Input: part model. Units: mm. Frame: model coordinates. A direction names the side the tool comes from. Coordinates: 2 decimals unless noted, no trailing zeros. Write each loop counter-clockwise with the first axis right and the second up, starting at its lowest first coordinate (ties: lowest second). Pieces come first, ordered by that corner, then holes. Notation, with made-up numbers: M 33.25,50.5 L 83.25,50.5 A13 cw 83.25,72.5 Z; hole C -8.75,1.25 d6. An arc over 180 degrees is marked long. Use one line per item in the form item = value.
from build123d import *

# Parameters (mm, degrees)
SKETCH_1_W           = 232.8
SKETCH_1_H           = 162
SKETCH_1_R           = 72
EXTRUDE_1_DEPTH      = 4
CUT_EXTRUDE_START    = -10
CUT_EXTRUDE_2_DEPTH  = 10
EXTRUDE_2_DEPTH      = 4
CUT_EXTRUDE_3_DEPTH  = 10
SKETCH_5_R           = 1.6
CUT_EXTRUDE_4_DEPTH  = 10
SKETCH_9_R           = 1.6
CUT_EXTRUDE_5_DEPTH  = 10
SKETCH_10_R          = 1.6
CUT_EXTRUDE_6_DEPTH  = 10
SKETCH_11_R          = 1.6
CUT_EXTRUDE_7_DEPTH  = 10
CUT_EXTRUDE_8_DEPTH  = 10
FILLET_1_R           = 3
FILLET_2_R           = 1.1
FILLET_3_R           = 3
CUT_EXTRUDE_9_DEPTH  = 10
FILLET_4_R           = 3
SKETCH_14_W          = 34.4
SKETCH_14_H          = 162
CUT_EXTRUDE_10_DEPTH = 10
CUT_EXTRUDE_11_DEPTH = 10
FILLET_5_R           = 3
SKETCH_16_R          = 1.55
CUT_EXTRUDE_12_DEPTH = 10
SKETCH_17_W          = 200
SKETCH_17_H          = 10
CUT_EXTRUDE_13_DEPTH = 5
FILLET_6_R           = 3


with BuildPart() as part:
    # 草图1 → 凸台-拉伸1 (new body)
    with BuildSketch(Plane.XY):
        Rectangle(SKETCH_1_W, SKETCH_1_H)
        Circle(SKETCH_1_R, mode=Mode.SUBTRACT)
    extrude(amount=EXTRUDE_1_DEPTH)

    # 草图3 → 切除-拉伸2 (cut)
    with BuildSketch(Plane.XY.offset(4).offset(CUT_EXTRUDE_START)):
        with BuildLine():
            Line((-21.634615385, 68.67272688), (-116.4, 38.817895988))
            Line((-116.4, 38.817895988), (-116.4, -7.313954951))
            Line((-116.4, -7.313954951), (-71.680591647, 6.774421088))
            ThreePointArc((-71.680591647, 6.774421088), (-55.989124219, 45.268288781), (-21.634615385, 68.67272688))
        make_face()
    extrude(amount=CUT_EXTRUDE_2_DEPTH, mode=Mode.SUBTRACT)

    # 草图6 → 凸台-拉伸2 (add)
    with BuildSketch(Plane.XY.offset(4)):
        Polygon((-126.671662246, -16.840640315), (-116.4, -29.949880057), (-116.4, -7.313954951), (-128.474546862, -11.117913075), align=None)
        Polygon((-116.4, 38.817895988), (-116.4, 54.514482194), (-143.498585323, 36.571480592), (-141.695700708, 30.848753352), align=None)
    extrude(amount=-EXTRUDE_2_DEPTH)

    # 草图7 → 切除-拉伸3 (cut)
    with BuildSketch(Plane.XY.offset(4)):
        Polygon((-116.4, -29.949880057), (-76.4, -81), (-116.4, -81), align=None)
        Polygon((-116.4, 54.514482194), (-76.4, 81), (-116.4, 81), align=None)
    extrude(amount=-CUT_EXTRUDE_3_DEPTH, mode=Mode.SUBTRACT)

    # 草图5 → 切除-拉伸4 (cut)
    with BuildSketch(Plane.XY.offset(4)):
        with Locations((-115.25907459, -12.196774271)):
            Circle(SKETCH_5_R)
        with Locations((-131.485036128, 39.307770889)):
            Circle(SKETCH_5_R)
    extrude(amount=-CUT_EXTRUDE_4_DEPTH, mode=Mode.SUBTRACT)

    # 草图9 → 切除-拉伸5 (cut)
    with BuildSketch(Plane.XY.offset(4)):
        with Locations((-22.836538462, 72.487878374)):
            Circle(SKETCH_9_R)
        with Locations((72.487878374, 22.836538462)):
            Circle(SKETCH_9_R)
        with Locations((22.836538462, -72.487878374)):
            Circle(SKETCH_9_R)
        with Locations((-72.487878374, -22.836538462)):
            Circle(SKETCH_9_R)
    extrude(amount=-CUT_EXTRUDE_5_DEPTH, mode=Mode.SUBTRACT)

    # 草图10 → 切除-拉伸6 (cut)
    with BuildSketch(Plane.XY.offset(4)):
        with Locations((-93.229198124, 50.99070111)):
            Circle(SKETCH_10_R)
    extrude(amount=-CUT_EXTRUDE_6_DEPTH, mode=Mode.SUBTRACT)

    # 草图11 → 切除-拉伸7 (cut)
    with BuildSketch(Plane(origin=(0, 0, 0), x_dir=(-1, 0, 0), z_dir=(0, 0, -1))):
        with Locations((-35.108799147, 67.404541557)):
            Circle(SKETCH_11_R)
        with Locations((-67.404541557, -35.108799147)):
            Circle(SKETCH_11_R)
        with Locations((35.108799147, -67.404541557)):
            Circle(SKETCH_11_R)
    extrude(amount=-CUT_EXTRUDE_7_DEPTH, mode=Mode.SUBTRACT)

    # 草图12 → 切除-拉伸8 (cut)
    with BuildSketch(Plane.XY.offset(4)):
        Polygon((-93.668674526, 62.369689763), (-74.593630829, 75), (-25.836538462, 75), (-25.836538462, 72.5912113), (-90.473635724, 52.227978291), align=None)
    extrude(amount=-CUT_EXTRUDE_8_DEPTH, mode=Mode.SUBTRACT)

    # 圆角1
    # the kernel refuses this fillet: 3 mm, written as the material it adds along each edge
    with BuildSketch(Plane(origin=(-25.836538462, 75, 4), x_dir=(0, -1, 0), z_dir=(0, 0, -1)), Plane(origin=(-90.473635724, 52.227978291, 4), x_dir=(-0.3004807692307691, 0.95378787333583, 0), z_dir=(0, 0, -1))) as fillet_1_piece_1:
        with BuildLine():
            CenterArc((FILLET_1_R, FILLET_1_R), FILLET_1_R, 180, 90)
            Line((0, FILLET_1_R), (0, 0))
            Line((0, 0), (FILLET_1_R, 0))
        make_face()
    extrude(amount=4)
    with BuildSketch(Plane(origin=(-25.836538462, 72.5912113, 4), x_dir=(-0.9537878733358296, -0.30048076923076983, 0), z_dir=(0, 0, -1))) as fillet_1_piece_2:
        with BuildLine():
            CenterArc((FILLET_1_R * 0.733411747334, FILLET_1_R), FILLET_1_R, 197.486481518, 72.513518482)
            Line((-FILLET_1_R * 0.220376126002, FILLET_1_R * 0.699519230769), (0, 0))
            Line((0, 0), (FILLET_1_R * 0.733411747334, 0))
        make_face()
    extrude(amount=4)
    with BuildSketch(Plane(origin=(-93.668674526, 62.369689763, 4), x_dir=(0.3004807692307694, -0.95378787333583, 0), z_dir=(0, 0, -1))) as fillet_1_piece_3:
        with BuildLine():
            CenterArc((FILLET_1_R * 0.753231578374, -FILLET_1_R), FILLET_1_R, 90, 73.976427328)
            Line((-FILLET_1_R * 0.207916633287, -FILLET_1_R * 0.72396718452), (0, 0))
            Line((0, 0), (FILLET_1_R * 0.753231578374, 0))
        make_face()
    extrude(amount=4)
    with BuildSketch(Plane(origin=(-74.593630829, 75, 4), x_dir=(1, 0, 0), z_dir=(0, 0, -1))) as fillet_1_piece_4:
        with BuildLine():
            CenterArc((FILLET_1_R * 0.30106152849, FILLET_1_R), FILLET_1_R, 236.48994581, 33.51005419)
            Line((-FILLET_1_R * 0.251021777541, FILLET_1_R * 0.166211043968), (0, 0))
            Line((0, 0), (FILLET_1_R * 0.30106152849, 0))
        make_face()
    extrude(amount=4)

    # 圆角2
    fillet_2_edges = [part.edges().sort_by_distance(p)[0] for p in [
        (-26.180986438, 73.395723271, 2),
    ]]
    fillet(fillet_2_edges, radius=FILLET_2_R)

    # 圆角3
    fillet_3_edges = [part.edges().sort_by_distance(p)[0] for p in [
        (-71.680591647, 6.774421088, 2),
        (-76.4, -81, 2),
        (-76.4, 81, 2),
    ]]
    fillet(fillet_3_edges, radius=FILLET_3_R)

    # 草图13 → 切除-拉伸9 (cut)
    with BuildSketch(Plane.XY.offset(4)):
        with BuildLine():
            Line((-71.696957036, -36.822633688), (-92.944059946, -46.914680662))
            Line((-92.944059946, -46.914680662), (-72.505072248, -73))
            Line((-72.505072248, -73), (-34.166650407, -73))
            ThreePointArc((-34.166650407, -73), (-55.937253271, -58.029162466), (-71.696957036, -36.822633688))
        make_face()
        with BuildLine():
            Line((-80.417945117, -5.414250016), (-116.543877682, -16.79534251))
            Line((-116.543877682, -16.79534251), (-96.104889984, -42.880661848))
            Line((-96.104889984, -42.880661848), (-73.842184412, -32.306219235))
            ThreePointArc((-73.842184412, -32.306219235), (-78.293303626, -19.144675692), (-80.417945117, -5.414250016))
        make_face()
    extrude(amount=-CUT_EXTRUDE_9_DEPTH, mode=Mode.SUBTRACT)

    # 圆角4
    fillet_4_edges = [part.edges().sort_by_distance(p)[0] for p in [
        (-80.417945117, -5.414250016, 2),
        (-73.842184412, -32.306219235, 2),
        (-96.104889984, -42.880661848, 2),
        (-116.543877682, -16.79534251, 2),
        (-71.696957036, -36.822633688, 2),
        (-34.166650407, -73, 2),
        (-72.505072248, -73, 2),
        (-92.944059946, -46.914680662, 2),
    ]]
    fillet(fillet_4_edges, radius=FILLET_4_R)

    # 草图14 → 切除-拉伸10 (cut)
    with BuildSketch(Plane.XY.offset(4)):
        with Locations((99.2, 0)):
            Rectangle(SKETCH_14_W, SKETCH_14_H)
    extrude(amount=-CUT_EXTRUDE_10_DEPTH, mode=Mode.SUBTRACT)

    # 草图15 → 切除-拉伸11 (cut)
    with BuildSketch(Plane.XY.offset(4)):
        with BuildLine():
            Line((32.726136344, 73), (74, 73))
            Line((74, 73), (74, 30.397368307))
            ThreePointArc((74, 30.397368307), (57.457489516, 55.665401269), (32.726136344, 73))
        make_face()
        with BuildLine():
            Line((74, -73), (74, -30.397368307))
            ThreePointArc((74, -30.397368307), (57.457489516, -55.665401269), (32.726136344, -73))
            Line((32.726136344, -73), (74, -73))
        make_face()
    extrude(amount=-CUT_EXTRUDE_11_DEPTH, mode=Mode.SUBTRACT)

    # 圆角5
    fillet_5_edges = [part.edges().sort_by_distance(p)[0] for p in [
        (82, 81, 2),
        (82, -81, 2),
        (74, 30.397368307, 2),
        (32.726136344, 73, 2),
        (74, 73, 2),
        (32.726136344, -73, 2),
        (74, -30.397368307, 2),
        (74, -73, 2),
    ]]
    fillet(fillet_5_edges, radius=FILLET_5_R)

    # 草图16 → 切除-拉伸12 (cut)
    with BuildSketch(Plane(origin=(0, 0, 0), x_dir=(-1, 0, 0), z_dir=(0, 0, -1))):
        with Locations((108.877259832, -33.065343142)):
            Circle(SKETCH_16_R)
        with Locations((85.167293187, -63.325259168)):
            Circle(SKETCH_16_R)
    extrude(amount=-CUT_EXTRUDE_12_DEPTH, mode=Mode.SUBTRACT)

    # 草图17 → 切除-拉伸13 (cut, symmetric)
    with BuildSketch(Plane.XY.offset(4)):
        with Locations((0, 83)):
            Rectangle(SKETCH_17_W, SKETCH_17_H)
        with Locations((0, -83)):
            Rectangle(SKETCH_17_W, SKETCH_17_H)
    extrude(amount=CUT_EXTRUDE_13_DEPTH, both=True, mode=Mode.SUBTRACT)

    # 圆角6
    fillet_6_edges = [part.edges().sort_by_distance(p)[0] for p in [
        (82, -78, 2),
        (82, 78, 2),
        (-80.930777947, 78, 2),
        (-78.750631108, -78, 2),
    ]]
    fillet(fillet_6_edges, radius=FILLET_6_R)


solid = part.part
(1) Line query: probe 1 along X at (y, z) = (-39.5, 3.1); probe 2 along Y at (x, z) = (3, 0.5); probe 3 along X at (y, z) = (-50, 2). Output: solid intervals per line, ascending.
Computed:
probe_1 = -108.92 to -98.75, -88.99 to -77.33, -70.26 to -60.2, 60.2 to 82
probe_2 = -78 to -71.94, 71.94 to 78
probe_3 = -100.69 to -90.53, -63.22 to -51.81, 51.81 to 62.45, 74 to 82
(2) Set-up query: faces 1 (the flat face through (-55, -47, 0)), 2 (the flat face through (-57.36, 62.66, 2.03)). Return all of +Z, -Z, +X, -X, +Y, -Y with unobstructed straight access to the full face (end or side cutting, diameter ignored); none if empty.
Computed:
face_1 = -Z, +X, -X, +Y, -Y
face_2 = +Z, -Z
(3) Section query B-B on x = -48. Return the cut outline in (y, z), plus the area to 3 significant figures.
Computed:
outline = M -78,0 L -73,0 L -73,4 L -78,4 Z; M -64.75,0 L -53.67,0 L -53.67,4 L -64.75,4 Z; M 60.37,0 L 65.61,0 L 65.61,4 L 60.37,4 Z; M 75,0 L 78,0 L 78,4 L 75,4 Z
area = 97.3 mm^2
(4) Section query A-A on x = 0. Return the cut outline in (y, z).
Computed:
outline = M -78,0 L -72,0 L -72,4 L -78,4 Z; M 72,0 L 78,0 L 78,4 L 72,4 Z
(5) First-contact query: pin 1 Ø3 at (x, y) = (-35.11, -67.4) entering from +Z; pin 2 Ø1.2 at (y, z) = (50, 3) entering from -X; pin 3 Ø5 at (x, y) = (72.49, 22.84) entering from +Z; pin 4 Ø2 at (y, z) = (-55, 1) entering from -X. Flat tips, straight axial feed; report the tip coordinate or a pass-through.
Computed:
pin_1 = through
pin_2 = -124.12
pin_3 = 4
pin_4 = -97.56
(6) Pull-direction query (X, two-part tool) for faces 3 (the flat face through (-55, -47, 4)), 4 (the flat face through (-105.843, -30.453, 2.028)); classes: pulls with the +X half, pulls with the -X half, needs draft (parallel to the pull), parting line crosses it, or undercut.
Computed:
face_3 = needs draft
face_4 = undercut
(7) Section query C-C on y = 0. Return the cut outline in (x, z), plus the area to 3 significant figures.
Computed:
outline = M -93.18,0 L -72,0 L -72,4 L -93.18,4 Z; M 72,0 L 82,0 L 82,4 L 72,4 Z
area = 125 mm^2
(8) Section query D-D on z = 3.1. State how many separate pieces and enclosed holes the cut face has, plus the area to 3 significant figures.
Computed:
separate_pieces = 1
enclosed_holes = 17
area = 7,380 mm^2
